Could you check a few things on this model? Use its own coordinates, in mm. A direction names the side the tool comes from. Round coordinates to 2 decimals unless told otherwise and drop trailing zeros. Loops run counter-clockwise (first coordinate to the right, second up) from the corner with the lowest first, then second, coordinate; pieces in that order, holes last. Notation, with made-up numbers: (-10, 86.5) -> (16, 86.5) arc R28 ccw to (16, 120.5) -> close; hole circle Ø8 at (31.5, 21.5). An arc over 180 degrees is marked (long way). Write each question's results on one line, items separated by ' | '. Start each with the question number.
1) Imagine slicing it at D-D, the plane z = 43.5. List the corners of the cut face in (x, y) for me, plus the area to 3 significant figures.
2) If I drill on probe 1 along Y at (x, z) = (13.25, 45); probe 2 along Z at (x, y) = (14, -27); probe 3 along Y at (x, z) = (7.5, -15.5), over which ranges is the centre line in solid material (lowest first)?
3) Imagine slicing it at A-A, the plane x = 2.25. List the corners of the cut face in (y, z) for me, plus the area to 3 significant figures.
4) Which directions (+Z, -Z, +X, -X, +Y, -Y) give clear straight access to the entire face, cutting with the end or side of a thin tool? Please do faces 1 (the flat face through (5, 0.076, -25)), 2 (the flat face through (18, -21, 47.156)), 3 (the flat face through (19, -21, 31.916)).
5) Imagine slicing it at B-B, the plane z = -45. List the corners of the cut face in (x, y) for me, plus the area to 3 significant figures.
6) We'd pull the mould along Y, two halves only. Please class faces 4 (the cylindrical face through (22.68, -13.72, 39.43)), 5 (the flat face through (19, -38.025, 40)), 6 (the flat face through (0, -26, -3)): pulls with the +Y half, pulls with the -Y half, needs draft (parallel to the pull), parting line crosses it, or undercut.
7) Imagine slicing it at C-C, the plane x = 18. List the corners of the cut face in (y, z) for me.
8) For P1, Ø4.5, axis at x = 18.5, y = -19, coming from the +Z side; P2, Ø12, axis at x = 21.5, z = 37, coming from the -Y side; P3, Ø5, axis at x = 21.5, y = -16, coming from the -Z side; P4, Ø4.5, axis at x = 19.05, y = -12.57, coming from the -Z side (3 decimals), each with a flat end and sliding along its axis, tell me the tip position at first contact or that it passes through.
from build123d import *

# Parameters (mm, degrees)
F1_DEPTH   = 25.4
F3_DEPTH   = 25.4
F1_FACE1_W = 25.4
F1_FACE1_H = 38.1020354138
F4_DEPTH   = 76.2
F5_DEPTH   = 25.4
F6_R       = 3.81
F7_DEPTH   = 25.4


with BuildPart() as f1:
    # F0 (on Right) → F1 (new body)
    with BuildSketch(Plane.YZ):
        Polygon((-3.7335716031, 66.174152714), (-38.0235716031, 66.5286004045), (-65.2428203725, 39.8663124475), (-17.6430062947, -113.8280024187), (-4.9430062947, -113.8280024187), (-4.9430062947, -50.8290516523), (-4.9430062947, -35.4195966316), (-4.783722371, -35.4195966316), (-4.0876944394, 31.9155797899), (-38.02458931, 31.9155797899), (-38.02458931, 47.1555797899), (-3.9301621325, 47.1555797899), align=None)
        Polygon((0.0764283969, 31.9155797899), (-4.0876944394, 31.9155797899), (-4.783722371, -35.4195966316), (0.0764283969, -35.4195966316), align=None)
        Polygon((-4.9430062947, -50.8290516523), (-4.9430062947, -113.8280024187), (0.0764283969, -113.8280024187), (0.0764283969, -35.4195966316), (-4.783722371, -35.4195966316), align=None)
        Polygon((0.0764283969, 66.1347696372), (-3.7335716031, 66.174152714), (-3.9301621325, 47.1555797899), (0.0764283969, 47.1555797899), align=None)
        Polygon((0.0764283969, 47.1555797899), (-3.9301621325, 47.1555797899), (-4.0876944394, 31.9155797899), (0.0764283969, 31.9155797899), align=None)
    extrude(amount=F1_DEPTH)

    # F0 (on Right) → F3 (join)
    with BuildSketch(Plane.YZ):
        Polygon((-4.0876944394, 31.9155797899), (-3.9301621325, 47.1555797899), (-38.02458931, 47.1555797899), (-38.02458931, 31.9155797899), align=None)
    extrude(amount=F3_DEPTH)

    # F2 (on face) + F1_face1 (on face) → F4 (cut)
    with BuildSketch(Plane(origin=(0, 0.0764283969, 0), x_dir=(-1, 0, 0), z_dir=(0, 1, 0))):
        Polygon((-12.7, 55.3310290966), (-3.81, 66.1347696372), (-12.7, 66.1347696372), align=None)
        with BuildLine():
            ThreePointArc((-12.7, -113.8280024187), (-22.1716577551, -37.2233399355), (-25.4, 39.8971140385))
            Line((-25.4, 39.8971140385), (-25.4, -113.8280024187))
            Line((-25.4, -113.8280024187), (-12.7, -113.8280024187))
        make_face()
        Polygon((-12.7, 55.3310290966), (-12.7, 66.1347696372), (-25.4, 66.1347696372), (-25.4, 39.8971140385), align=None)
        Polygon((-12.7, 39.8971140385), (-3.81, 66.1347696372), (-12.7, 55.3310290966), align=None)
        Polygon((-25.4, 39.8971140385), (-12.7, 39.8971140385), (-12.7, 55.3310290966), align=None)
        with BuildLine():
            ThreePointArc((-3.81, -113.8280024187), (-10.5684247316, -37.0992306938), (-12.7, 39.8971140385))
            Line((-12.7, 39.8971140385), (-25.4, 39.8971140385))
            ThreePointArc((-25.4, 39.8971140385), (-22.1716577551, -37.2233399355), (-12.7, -113.8280024187))
            Line((-12.7, -113.8280024187), (-3.81, -113.8280024187))
        make_face()
    with BuildSketch(Plane(origin=(12.7, -18.9735716031, 66.3316850209), x_dir=(1, 0, 0), z_dir=(0, 0.0103362134, 0.9999465799))):
        Rectangle(F1_FACE1_W, F1_FACE1_H)
    extrude(amount=-F4_DEPTH, dir=(0, 1, 0), mode=Mode.SUBTRACT)

    # F0 (on Right) → F5 (join)
    with BuildSketch(Plane.YZ):
        Polygon((-4.0876944394, 31.9155797899), (-3.9301621325, 47.1555797899), (-38.02458931, 47.1555797899), (-38.02458931, 31.9155797899), align=None)
    extrude(amount=F5_DEPTH)

    # F6 (on face) → F7 (cut)
    with BuildSketch(Plane(origin=(0, 0, 31.9155797899), x_dir=(1, 0, 0), z_dir=(0, 0, -1))):
        with Locations((19.0471851579, 12.5712944394)):
            Circle(F6_R)
        with Locations((19.0471851579, 29.54098931)):
            Circle(F6_R)
    extrude(amount=-F7_DEPTH, mode=Mode.SUBTRACT)


solid = f1.part
Checked values:
1) outline: (0, -61.53) -> (11.48, -61.53) -> (11.48, -38.02) -> (25.4, -38.02) -> (25.4, -3.97) -> (11.48, -3.97) -> (11.48, 0.08) -> (0, 0.08) -> close; hole circle Ø7.62 at (19.05, -29.54); hole circle Ø7.62 at (19.05, -12.57) | area: 1,090 mm^2
2) probe 1: -38.02 to -3.95 | probe 2: 31.92 to 47.16 | probe 3: -48.1 to 0.08
3) outline: (-65.24, 39.87) -> (-17.64, -113.83) -> (0.08, -113.83) -> (0.08, 66.13) -> (-38.43, 66.13) -> close; hole (-4.94, -50.83) -> (-4.78, -35.42) -> (-4.94, -35.42) -> close | area: 7,740 mm^2
4) face 1: +Z, -Z, +X, -X, +Y | face 2: +Z, +X, +Y, -Y | face 3: -Z, +X, +Y, -Y
5) outline: (0, -38.96) -> (10.09, -38.96) -> (10.09, -4.94) -> (0, -4.94) -> close; (0, -4.88) -> (10.09, -4.88) -> (10.09, 0.08) -> (0, 0.08) -> close | area: 393 mm^2
6) face 4: undercut | face 5: pulls with the -Y half | face 6: needs draft
7) outline: (-38.02, 31.92) -> (-33.2, 31.92) -> (-33.2, 47.16) -> (-38.02, 47.16) -> close; (-25.88, 31.92) -> (-16.23, 31.92) -> (-16.23, 47.16) -> (-25.88, 47.16) -> close; (-8.91, 31.92) -> (-4.09, 31.92) -> (-3.93, 47.16) -> (-8.91, 47.16) -> close
8) P1: z = 47.16 | P2: y = -38.02 | P3: z = 31.92 | P4: through
